The listing builds one solid part. Answer for the finished solid, in the listing's coordinates (mm). A direction names the side the tool comes from. Coordinates: 2 decimals unless noted, no trailing zeros. Order: outer loops, then holes, each group sorted by start corner. A loop starts at its lowest first (then second) coordinate and runs counter-clockwise, first axis right, second up. Notation, with made-up numbers: (-15.75, -22.75) -> (1.25, -22.75) arc R17 cw to (1.25, 5.25) -> close; hole circle Ø9 at (52, 8.5). An arc over 180 degrees is marked (long way). Put each result on its own line as item: value. Start each with the question number.
```python
from build123d import *

# Parameters (mm, degrees)
F1_DEPTH = 150
F2_DEPTH = 5
F2_TAPER = -25
F3_SIZE  = 1


with BuildPart() as f1:
    # F0 (on Front) → F1 (new body)
    with BuildSketch(Plane.XZ):
        Polygon((6.776461585, 9.0722467188), (-5.5767488922, -3.059325051), (-3.258036708, -2.8919032872), (-8.1410452514, -8.8131905165), (-5.7786260987, -8.3639572937), (-12.4195150821, -17.3975064051), (2.255862786, -4.3973731032), (0.1915401989, -4.3973731032), (3.8383661048, 0.4654207636), (1.3486526159, 0.4654207636), align=None)
    extrude(amount=F1_DEPTH)

    # F1_face (on face) → F2 (join)
    with BuildSketch(Plane(origin=(-2.1628477345, 0, -4.133992699), x_dir=(1, 0, 0), z_dir=(0, 1, 0))):
        Polygon((2.3543879334, 0.2633804043), (4.4187105205, 0.2633804043), (-10.2566673476, 13.2635137061), (-3.6157783642, 4.2299645948), (-5.9781975168, 4.6791978175), (-1.0951889734, -1.2420894118), (-3.4139011576, -1.074667648), (8.9393093195, -13.2062394177), (3.5115003504, -4.5994134625), (6.0012138393, -4.5994134625), align=None)
    extrude(amount=F2_DEPTH, taper=F2_TAPER)

    # F3
    f3_edges = [f1.edges().sort_by_distance(p)[0] for p in [
        (-5.081826, -150, -10.89744),
        (2.014953, -150, -1.965976),
        (1.223701, -150, -4.397373),
        (2.593509, -150, 0.465421),
        (4.062557, -150, 4.768834),
        (0.599856, -150, 3.006461),
        (-4.417393, -150, -2.975614),
        (-5.699541, -150, -5.852547),
        (-6.959836, -150, -8.588574),
        (-9.099071, -150, -12.880732),
    ]]
    chamfer(f3_edges, length=F3_SIZE)


solid = f1.part
```
(1) Find the intervals of material crossed by L1, parallel to Z at x = 1, y = -104.5; L2, parallel to Z at x = -2, y = -83.5; L3, parallel to Z at x = -4.5, y = -136.5, in increasing order.
(2) For a pull along Z with two mould halves and no side action, classify faces 1 (the flat face through (0.686, -73.457, 3.091)), 2 (the flat face through (-2, -150, -4)), 3 (the flat face through (-4.532, -149.493, -5.211)), 4 (the flat face through (-3.816, -149.396, -9.248)) as released by +Z, released by -Z, zero draft, split by the parting line, or undercut.
(3) The part is cut by section A-A on y = -62. Determine the outline of the cut face in (x, z), plus the area to 3 significant figures.
(4) Each of these flat-tipped pins is pushed along its axis until it touches: P1, Ø4, axis at x = -10, y = -102, coming from the -Z side; P2, Ø1.7, axis at x = 1, y = -100.5, coming from the +Z side; P3, Ø5, axis at y = -54.5, z = -12, coming from the -X side. Where does it stop, or does it pass through?
(5) A tool of negligible diameter and unlimited length cuts with its end or side. For faces 5 (the flat face through (-5.2, -73.5, -11)), 6 (the flat face through (4.025, -73.457, 4.709)), 7 (the flat face through (-3, 5, -5)), from which of +Z, -Z, +X, -X, +Y, -Y can it reach the whole face along a straight path? Write none if from no direction.
Worked out:
1. L1: -5.51 to -4.4, -3.32 to 3.4
1. L2: -8.17 to 0.45
1. L3: -10.38 to -4.4, -2.98 to -2
2. face 1: released by +Z
2. face 2: zero draft
2. face 3: undercut
2. face 4: released by -Z
3. outline: (-12.42, -17.4) -> (2.26, -4.4) -> (0.19, -4.4) -> (3.84, 0.47) -> (1.35, 0.47) -> (6.78, 9.07) -> (-5.58, -3.06) -> (-3.26, -2.89) -> (-8.14, -8.81) -> (-5.78, -8.36) -> close
3. area: 83.5 mm2
4. P1: z = -17.03
4. P2: z = 4.23
4. P3: x = -10.29
5. face 5: -Z, +X, -Y
5. face 6: +X, -Y
5. face 7: +Z, -Z, +X, -X, +Y
